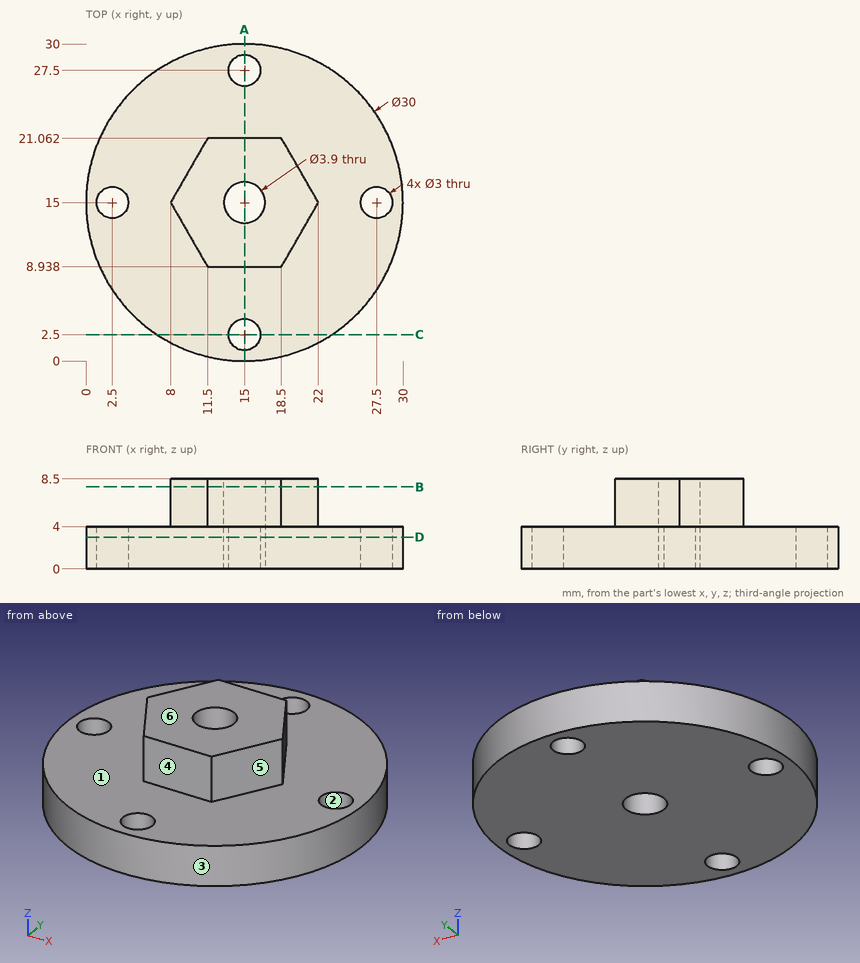
Geometry check sheet. Reference: drawing and pictorial views, mm from the part's lowest x, y, z. A direction names the side the tool comes from. Coordinates: 2 decimals unless noted, no trailing zeros. Order: outer loops, then holes, each group sorted by start corner. A loop starts at its lowest first (then second) coordinate and runs counter-clockwise, first axis right, second up. Notation, with made-up numbers: (44, 29.25) - (68, 29.25) arc R23 cw to (68, 44.25) - close; hole circle Ø1 at (22.25, -35.5). An arc over 180 degrees is marked (long way). One line per item, written item: value.
(1) Sectioned sample at B-B (z = 7.75). Enter the section's corners in (x, y).
Data:
outline: (8, 15) - (11.5, 8.94) - (18.5, 8.94) - (22, 15) - (18.5, 21.06) - (11.5, 21.06) - close; hole circle Ø3.9 at (15, 15)
(2) Sectioned sample at D-D (z = 3). Enter the section's corners in (x, y).
Data:
outline: circle Ø30 at (15, 15); hole circle Ø3 at (2.5, 15); hole circle Ø3.9 at (15, 15); hole circle Ø3 at (15, 2.5); hole circle Ø3 at (15, 27.5); hole circle Ø3 at (27.5, 15)
(3) Access from +Z, -Z, +X, -X, +Y, -Y to the whole of each face (thin tool, end or side, straight path). Record for the marked faces 4, 5 and 6.
Data:
face 4: +Z, +X, -X, -Y
face 5: +Z, +X, -Y
face 6: +Z, +X, -X, +Y, -Y
(4) Release check for a two-part mould opening along Y. For the marked faces 1, 2 and 3 record: +Y half, -Y half, draft (parallel to the pull), parting line (faces both ways), or undercut.
Data:
face 1: draft
face 2: undercut
face 3: parting line
(5) Sectioned sample at C-C (y = 2.5). Enter the section's corners in (x, z), and give its area (3 significant figures).
Data:
outline: (6.71, 0) - (13.5, 0) - (13.5, 4) - (6.71, 4) - close; (16.5, 0) - (23.29, 0) - (23.29, 4) - (16.5, 4) - close
area: 54.3 mm^2
(6) Sectioned sample at A-A (x = 15). Enter the section's corners in (y, z).
Data:
outline: (0, 0) - (1, 0) - (1, 4) - (0, 4) - close; (4, 0) - (13.05, 0) - (13.05, 8.5) - (8.94, 8.5) - (8.94, 4) - (4, 4) - close; (16.95, 0) - (26, 0) - (26, 4) - (21.06, 4) - (21.06, 8.5) - (16.95, 8.5) - close; (29, 0) - (30, 0) - (30, 4) - (29, 4) - close
(7) Thickness scan on probe 1 along Y at (x, z) = (15, 2.25); probe 2 along Y at (x, z) = (15, 5); probe 3 along Y at (x, z) = (14.25, 3.75). Record the ranges inside material, lowest first. Write a range as from..to.
Data:
probe 1: y = 0..1, 4..13.05, 16.95..26, 29..30
probe 2: y = 8.94..13.05, 16.95..21.06
probe 3: y = 0.02..1.2, 3.8..13.2, 16.8..26.2, 28.8..29.98
(8) Depth check by flat-ended pin: pin 1 Ø2 at (y, z) = (18, 1) entering from +X; pin 2 Ø1.8 at (x, y) = (15, 27.5) entering from -Z; pin 3 Ø1 at (y, z) = (13, 5.5) entering from +X; pin 4 Ø2 at (x, z) = (15.5, 5.5) entering from -Y. Enter the tip coordinate at first touch or a pass-through.
Data:
pin 1: stops at x = 29.87
pin 2: passes through
pin 3: stops at x = 21.13
pin 4: stops at y = 8.94
